Part print with two shaded views. Sizes in mm from the minimum x, y, z corner. Coordinates: 2 decimals unless noted, no trailing zeros. Loops run counter-clockwise (first coordinate to the right, second up) from the corner with the lowest first, then second, coordinate; pieces in that order, holes last.
Item 1: Flat gauge pins, fed straight in: pin 1 (2 mm diameter, centred on x = 34.67, z = 4.62, fed in from +Y); pin 2 (5.5 mm diameter, centred on x = 34.67, z = 4.62, fed in from -Y). Where does each tip first touch, or does it go through?
Item 2: Cut at A-A (y = 3.25). List the corners of the cut face in (x, z) (1 decimal).
Item 3: Drill centre lines: line 1 along X through (y, z) = (4, 4.5); line 2 along Z through (x, y) = (6, 0.8) (1 decimal); line 3 along X through (y, z) = (3.25, 45) (1 decimal). Where is each one in solid material? Low to high.
Item 4: Cut at B-B (z = 4). Count the separate pieces of the cut face and the enclosed holes in it, and give its area (3 significant figures).
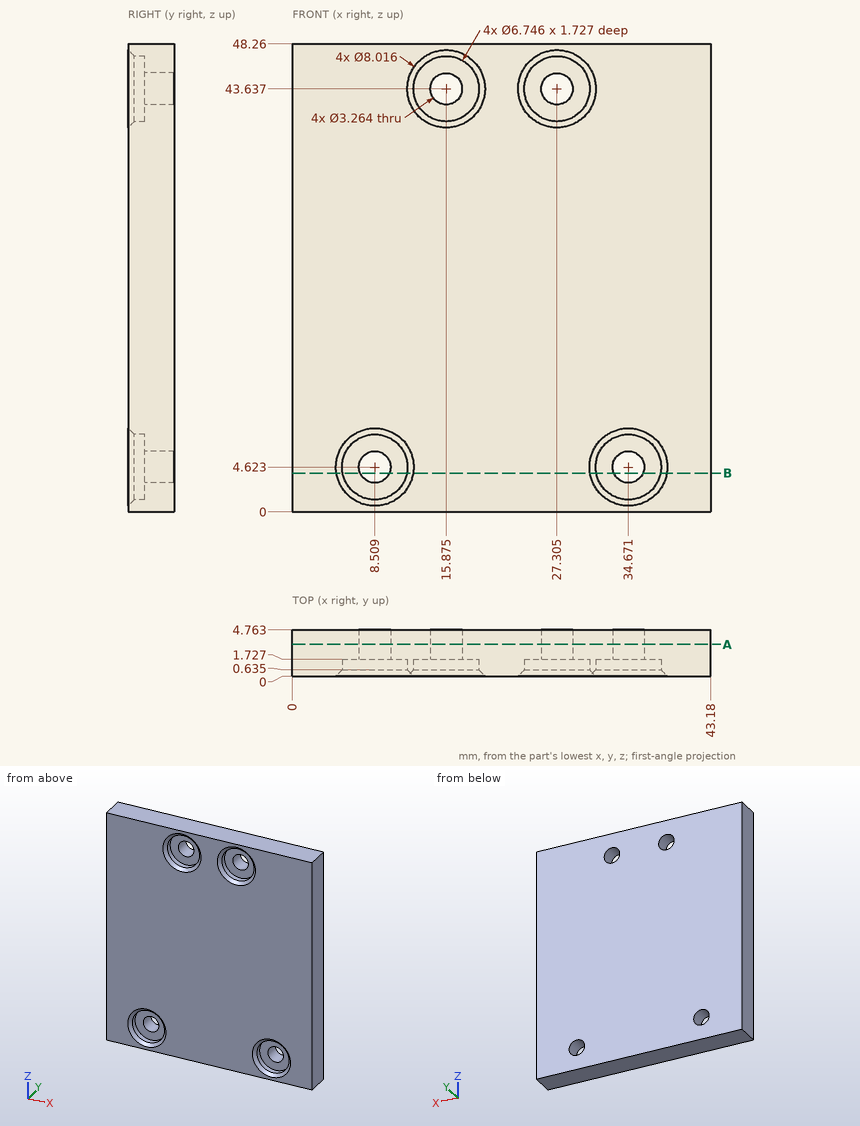
Filled sheet:
1. pin 1: passes through
1. pin 2: stops at y = 1.73
2. outline: (0, 0) - (43.2, 0) - (43.2, 48.3) - (0, 48.3) - close; hole circle Ø3.3 at (8.5, 4.6); hole circle Ø3.3 at (15.9, 43.6); hole circle Ø3.3 at (27.3, 43.6); hole circle Ø3.3 at (34.7, 4.6)
3. line 1: x = 0 to 6.88, 10.14 to 33.04, 36.3 to 43.18
3. line 2: z = 0 to 2.4, 6.9 to 48.3
3. line 3: x = 0 to 15, 16.8 to 26.4, 28.2 to 43.2
4. separate pieces: 3
4. enclosed holes: 0
4. area: 164 mm2
